Could you check a few things on this model? Use its own coordinates, in mm. Face numbers are marked on the shaded views. A direction names the side the tool comes from. Coordinates: 2 decimals unless noted, no trailing zeros. Write each loop counter-clockwise with the first axis right and the second up, starting at its lowest first coordinate (ties: lowest second). Pieces come first, ordered by that corner, then holes.
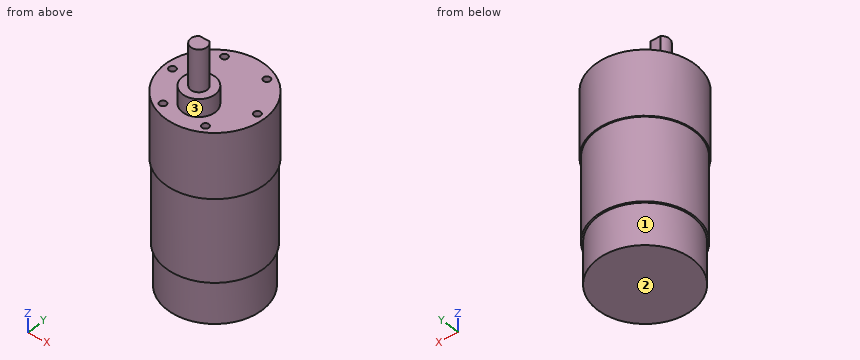
```python
from build123d import *

# Parameters (mm, degrees)
SKETCH1_R                       = 17.4
BOSS_EXTRUDE1_DEPTH             = 15.4
SKETCH2_R                       = 18
BOSS_EXTRUDE2_DEPTH             = 30.7
SKETCH3_R                       = 18.4
BOSS_EXTRUDE3_DEPTH             = 24
SKETCH4_R                       = 6
BOSS_EXTRUDE4_DEPTH             = 6.5
SKETCH5_R                       = 3
BOSS_EXTRUDE5_DEPTH             = 15.5
CUT_EXTRUDE1_DEPTH              = 13
TAP_DRILL_FOR_M3X0_5_TAP1_D     = 2.5
TAP_DRILL_FOR_M3X0_5_TAP1_DEPTH = 10.76


with BuildPart() as part:
    # Sketch1 → Boss-Extrude1 (new body)
    with BuildSketch(Plane.XY):
        Circle(SKETCH1_R)
    extrude(amount=BOSS_EXTRUDE1_DEPTH)

    # Sketch2 → Boss-Extrude2 (add)
    with BuildSketch(Plane.XY.offset(15.4)):
        Circle(SKETCH2_R)
    extrude(amount=BOSS_EXTRUDE2_DEPTH)

    # Sketch3 → Boss-Extrude3 (add)
    with BuildSketch(Plane.XY.offset(46.1)):
        Circle(SKETCH3_R)
    extrude(amount=BOSS_EXTRUDE3_DEPTH)

    # Sketch4 → Boss-Extrude4 (add)
    with BuildSketch(Plane.XY.offset(70.1)):
        with Locations((0, -7)):
            Circle(SKETCH4_R)
    extrude(amount=BOSS_EXTRUDE4_DEPTH)

    # Sketch5 → Boss-Extrude5 (add)
    with BuildSketch(Plane.XY.offset(76.6)):
        with Locations((0, -7)):
            Circle(SKETCH5_R)
    extrude(amount=BOSS_EXTRUDE5_DEPTH)

    # Sketch6 → Cut-Extrude1 (cut)
    with BuildSketch(Plane.XY.offset(92.1)):
        with BuildLine():
            Line((-1.8, -4.6), (1.8, -4.6))
            ThreePointArc((1.8, -4.6), (0, -4), (-1.8, -4.6))
        make_face()
    extrude(amount=-CUT_EXTRUDE1_DEPTH, mode=Mode.SUBTRACT)

    # Tap Drill for M3x0.5 Tap1
    with Locations(Plane.XY.offset(70.1)):
        with Locations((-15.5, 0), (-7.75, 13.423393759), (7.75, 13.423393759), (15.5, 0), (7.75, -13.423393759), (-7.75, -13.423393759)):
            Hole(TAP_DRILL_FOR_M3X0_5_TAP1_D / 2, depth=TAP_DRILL_FOR_M3X0_5_TAP1_DEPTH)


solid = part.part
```
1. For pin 1 (0.8 mm diameter, centred on x = -7, y = -13.5, fed in from +Z); pin 2 (3 mm diameter, centred on x = -15.5, y = 0, fed in from +Z); pin 3 (1 mm diameter, centred on y = -7, z = 48.5, fed in from +X), each with a flat end and sliding along its axis, tell me the tip position at first contact or that it passes through.
Verdict:
pin 1: stops at z = 59.34
pin 2: stops at z = 70.1
pin 3: stops at x = 17.21
2. I want a section at C-C on z = 65.5. Please give me the cut outline in (x, y), plus the area to 3 significant figures.
Verdict:
outline: circle Ø36.8 at (0, 0); hole circle Ø2.5 at (-15.5, 0); hole circle Ø2.5 at (-7.75, -13.42); hole circle Ø2.5 at (-7.75, 13.42); hole circle Ø2.5 at (7.75, -13.42); hole circle Ø2.5 at (7.75, 13.42); hole circle Ø2.5 at (15.5, 0)
area: 1,030 mm2
3. I want a section at B-B on y = 0. Please give me the cut outline in (x, z), plus the area to 3 significant figures.
Verdict:
outline: (-18.4, 46.1) - (-18, 46.1) - (-18, 15.4) - (-17.4, 15.4) - (-17.4, 0) - (17.4, 0) - (17.4, 15.4) - (18, 15.4) - (18, 46.1) - (18.4, 46.1) - (18.4, 70.1) - (16.75, 70.1) - (16.75, 59.34) - (14.25, 59.34) - (14.25, 70.1) - (-14.25, 70.1) - (-14.25, 59.34) - (-16.75, 59.34) - (-16.75, 70.1) - (-18.4, 70.1) - close
area: 2,470 mm2
4. I want a section at A-A on x = 0. Please give me the cut outline in (y, z).
Verdict:
outline: (-18.4, 46.1) - (-18, 46.1) - (-18, 15.4) - (-17.4, 15.4) - (-17.4, 0) - (17.4, 0) - (17.4, 15.4) - (18, 15.4) - (18, 46.1) - (18.4, 46.1) - (18.4, 70.1) - (-1, 70.1) - (-1, 76.6) - (-4, 76.6) - (-4, 79.1) - (-4.6, 79.1) - (-4.6, 92.1) - (-10, 92.1) - (-10, 76.6) - (-13, 76.6) - (-13, 70.1) - (-18.4, 70.1) - close
5. On a 3-axis mill with a long thin cutter (end or side, diameter ignored), from which of +Z, -Z, +X, -X, +Y, -Y can I reach the whole of each face in a straight line? I mean the marked faces 1, 2 and 3. Say none if no direction works.
Verdict:
face 1: -Z
face 2: -Z, +X, -X, +Y, -Y
face 3: +Z
6. I want a section at D-D on z = 85. Please give me the cut outline in (x, y), plus the area to 3 significant figures.
Verdict:
outline: (-1.8, -4.6) arc R3 ccw (long way) to (1.8, -4.6) - close
area: 26.8 mm2
7. Please list where these lines run through material, in increasing order: line 1 along Y through (x, z) = (7.75, 66.75); line 2 along Y through (x, z) = (7, 62); line 3 along Z through (x, y) = (-11.5, 0).
Verdict:
line 1: y = -16.69 to -14.67, -12.17 to 12.17, 14.67 to 16.69
line 2: y = -17.02 to -14.42, -12.42 to 12.42, 14.42 to 17.02
line 3: z = 0 to 70.1
